Autodesk Inventor part; units mm, degrees
ref_plane "Work Plane1" through (0, 304.8, 0) normal (0, 1, 0) x (-1, 0, 0)
ref_plane "Work Plane2" through (533.4, 247.5686, 0) normal (0, 1, 0) x (-1, 0, 0)
ref_plane "YZ Plane" through (0, 0, 0) normal (1, 0, 0) x (0, 1, 0)
sketch "Sketch1" plane through (0, 0, 0) normal (0, 0, 1) x (1, 0, 0)
  line L0 (0, 0) -> (0, -41.796)
  line L1 (25.4, -16.396) -> (25.4, -41.796)
  arc A0 (0, 0) -> (25.4, -16.396) centre (177.8, 247.5686) ccw
  line L2 (355.6, 0) -> (355.6, -41.796)
  line L3 (330.2, -16.396) -> (330.2, -41.796)
  arc A1 (330.2, -16.396) -> (355.6, 0) centre (177.8, 247.5686) ccw
  line L4 (177.8, 247.5686) -> (533.4, 247.5686)
  line L5 (25.4, -41.796) -> (0, -41.796)
  line L6 (330.2, -41.796) -> (331.8938, -41.796)
  line L7 (331.8938, -41.796) -> (355.6, -41.796)
revolve "Revolution1" add sketch "Sketch1" angle 110 about axis through (177.8, 247.5686, 0) along (1, 0, 0)
sketch "Sketch2" plane through (0, -41.796, 0) normal (0, 0, 1) x (1, 0, 0)
  line L0 (25.4, 0) -> (25.4, 25.4)
  line L1 (355.6, 41.796) -> (355.6, 0)
  arc A0 (330.2, 25.4) -> (355.6, 41.796) centre (177.8, 289.3645) ccw
  line L2 (330.2, 0) -> (330.2, 25.4)
  arc A1 (25.4, 25.4) -> (330.2, 25.4) centre (177.8, 289.3645) ccw
  arc A2 (25.4, 0) -> (330.2, 0) centre (177.8, 263.9645) ccw
  line L3 (25.4, 25.4) -> (25.4, 0)
  line L4 (330.2, 25.4) -> (330.2, 0)
  line L5 (177.8, 289.3645) -> (533.4, 289.3645)
  line L6 (355.6, 0) -> (330.2, 0)
  dimension "d6" = 304.8
  dimension "d7" = 304.8
revolve "Revolution2" add sketch "Sketch2" angle 4 about axis through (177.8, 247.5686, 0) along (1, 0, 0) contours L0 A1 L2 A2
ref_plane "Work Plane1" through (0, 304.8, 0) normal (0, 1, 0) x (-1, 0, 0)
ref_plane "Work Plane2" through (533.4, 247.5686, 0) normal (0, 1, 0) x (-1, 0, 0)
sketch "Sketch8" plane through (533.4, 247.5686, 0) normal (0, 1, 0) x (-1, 0, 0)
  arc A0 (177.8, -247.5686) -> (203.2, -263.9645) centre (355.6, 0) ccw
  line L0 (203.2, -263.9645) -> (203.2, -289.3645)
  line L1 (203.2, -289.3645) -> (177.8, -289.3645)
  line L2 (177.8, -289.3645) -> (177.8, -247.5686)
  line L3 (508, -289.3645) -> (508, -263.9645)
  line L4 (533.4, -247.5686) -> (533.4, -289.3645)
  line L5 (533.4, -289.3645) -> (508, -289.3645)
  arc A1 (203.2, -263.9645) -> (508, -263.9645) centre (355.6, 0) ccw
  arc A2 (203.2, -289.3645) -> (508, -289.3645) centre (355.6, -25.4) ccw
  line L6 (203.2, -289.3645) -> (203.2, -263.9645)
  line L7 (508, -263.9645) -> (508, -289.3645)
  line L8 (355.6, 0) -> (533.4, 0)
  arc A3 (508, -263.9645) -> (533.4, -247.5686) centre (355.6, 0) ccw
  dimension "d44" = 304.8
  dimension "d45" = 304.8
revolve "Revolution4" add sketch "Sketch8" angle 4 about axis through (177.8, 247.5686, 0) along (-1, 0, 0) contours A1 L3 A2 L0
sketch "Sketch9" plane through (25.4, 247.5686, -263.9645) normal (1, 0, 0) x (0, 0, -1)
  line L0 (0, 0) -> (25.4, 0)
  line L1 (-15.919, 90.2812) -> (7.9492, 98.9685)
  line L2 (-3.9849, 94.6248) -> (-3.9849, 81.9248)
  point P0 (-263.9645, -247.5686)
  dimension "d47" = 12.7
hole "Hole3" at (25.4, 329.4934, -259.9796) direction (1, 0, 0) diameter 6.35 end through all
hole "Hole4" at (25.4, 329.4934, -259.9796) direction (-1, 0, 0) diameter 6.35 end through all
sketch "Sketch10" plane through (355.6, -41.796, 0) normal (1, 0, 0) x (0, 0, -1)
  arc A0 (0, 0) -> (271.9137, 388.333) centre (0, 289.3645) ccw
  line L0 (237.0336, 123.3919) -> (467.2357, 16.0468)
  line L1 (165.9727, 52.331) -> (419.9727, 52.331) construction
  line L2 (279.5047, 214.4715) -> (509.7069, 107.1264)
  line L3 (237.0336, 123.3919) -> (491.0336, 123.3919) construction
  line L4 (509.7069, 107.1264) -> (467.2357, 16.0468)
  arc A1 (237.0336, 123.3919) -> (279.5047, 214.4715) centre (0, 289.3645) ccw
  dimension "d65" = 254
  dimension "d66" = 25
  dimension "d67" = 254
  dimension "d68" = 25
extrude "Extrusion3" add sketch "Sketch10" against normal blind 25.4
sketch "Sketch11" plane through (0, -41.796, 0) normal (-1, 0, 0) x (0, 0, 1)
  arc A0 (-271.9137, 388.333) -> (0, 0) centre (0, 289.3645) ccw
  line L0 (-279.5047, 214.4715) -> (-509.7069, 107.1264)
  line L1 (-509.7069, 107.1264) -> (-467.2357, 16.0468)
  line L2 (-467.2357, 16.0468) -> (-237.0336, 123.3919)
extrude "Extrusion4" add sketch "Sketch11" against normal blind 25.4
sketch "Sketch12" plane through (0, -41.796, 0) normal (-1, 0, 0) x (0, 0, 1)
  line L0 (-509.7069, 107.1264) -> (-467.2357, 16.0468)
  line L1 (-467.2357, 16.0468) -> (-237.0336, 123.3919)
  line L2 (-488.4713, 61.5866) -> (-350.35, 125.9937)
  dimension "d73" = 152.4
hole "Hole5" at (0, 84.1977, -350.35) direction (1, 0, 0) diameter 12.7 end through all
sketch "Sketch13" plane through (177.8, 247.5686, -25.4) normal (0, 1, 0) x (1, 0, 0)
  line L0 (152.4, 263.9645) -> (152.4, 238.5645)
  arc A0 (152.4, 238.5645) -> (-152.4, 238.5645) centre (0, -25.4) ccw
  line L1 (152.4, 263.9645) -> (152.4, 352.8645)
  line L2 (152.4, 352.8645) -> (76.2, 352.8645)
  line L3 (76.2, 279.4) -> (76.2, 269.7213)
  line L4 (119.5299, 269.7213) -> (119.5299, 257.7498)
  line L5 (119.5299, 257.7498) -> (152.4, 257.7498)
  line L6 (152.4, 263.9645) -> (152.4, 257.7498)
  line L7 (119.5299, 269.7213) -> (76.2, 269.7213)
  line L8 (-152.4, 238.5645) -> (-152.4, 263.9645)
  line L9 (76.2, 352.8645) -> (0, 352.8645)
  line L10 (0, 352.8645) -> (0, 279.4)
  line L11 (0, 279.4) -> (76.2, 279.4)
  point P0 (-177.8, -25.4)
  dimension "d81" = 88.9
  dimension "d82" = 76.2
  dimension "d85" = 76.2
extrude "Extrusion5" add sketch "Sketch13" against normal blind 18.288 contours L0 L5 L4 L7 L3 L11 L10 L9 L2 L1
sketch "Sketch14" plane through (355.6, -41.796, 0) normal (1, 0, 0) x (0, 0, -1)
  circle A0 centre (350.35, 125.9937) radius 6.35
  circle A1 centre (259.9796, 371.2894) radius 3.175
  line L0 (0, 41.796) -> (0, 0)
  arc A2 (0, 0) -> (237.0336, 123.3919) centre (0, 289.3645) ccw
  line L1 (237.0336, 123.3919) -> (467.2357, 16.0468)
  line L2 (467.2357, 16.0468) -> (509.7069, 107.1264)
  line L3 (509.7069, 107.1264) -> (279.5047, 214.4715)
  arc A3 (279.5047, 214.4715) -> (271.9137, 388.333) centre (0, 289.3645) ccw
  line L4 (232.6384, 374.038) -> (271.9137, 388.333)
  arc A4 (0, 41.796) -> (232.6384, 374.038) centre (0, 289.3645) ccw
  dimension "d86" = 272.5823
properties part number "Inner" material "Polystyrene"
Geometry check sheet. Reference: the model listing, model coordinates, mm. A direction names the side the tool comes from. Round coordinates to 2 decimals unless told otherwise and drop trailing zeros. Order: outer loops, then holes, each group sorted by start corner. A loop starts at its lowest first (then second) coordinate and runs counter-clockwise, first axis right, second up. Notation, with made-up numbers: M 25,7 L 55,7 A20 cw 55,15 Z; hole C -11,-20.75 d4. An arc over 180 degrees is marked long. Write item = value, one per line.
Q1. Depth check by flat-ended pin: pin 1 Ø4 at (y, z) = (329.49, -259.98) entering from +X; pin 2 Ø5.5 at (x, y) = (224, 237) entering from -Z; pin 3 Ø20 at (y, z) = (234.5, -337) entering from +X; pin 4 Ø5.5 at (y, z) = (242, -361.5) entering from -X. Enter the tip coordinate at first touch or a pass-through.
Answer block:
pin_1 = through
pin_2 = -378.26
pin_3 = 330.2
pin_4 = 177.8
Q2. Scan lines: line 1 (X direction, y = -32.5, z = -22.5); line 2 (Y direction, x = 7, z = -350); line 3 (Y direction, x = 256, z = -356). Record each from-to range of solid material in increasing order.
Answer block:
line_1 = 0 to 25.4, 330.2 to 355.6
line_2 = 28.92 to 77.86, 90.54 to 139.8
line_3 = 229.28 to 247.57
Q3. Set-up check for faces 1 (the flat face through (179.93, 225.85, -310.58)), 2 (the flat face through (175.666, -63.011, -21.718)), 3 (the flat face through (330.2, 298, -274)), 4 (the flat face through (12.52, 27.17, -353.75)): record each of +Z, -Z, +X, -X, +Y, -Y from which the full face is reachable in a straight line by a thin tool's end or side.
Answer block:
face_1 = +Z, -Y
face_2 = -Z, +Y
face_3 = +Z, -Z, +Y
face_4 = +X, -X, -Y
Q4. Release check for a two-part mould opening along Z. For faces 5 (the flat face through (12.522, 119.754, -392.994)), 6 (the flat face through (0, 96, -294)), 7 (the cylindrical face through (12.878, 79.906, -355.03)) record: released by +Z, released by -Z, zero draft, split by the parting line, or undercut.
Answer block:
face_5 = released by -Z
face_6 = zero draft
face_7 = undercut
Q5. Section check B-B (z = -419.5). Enter the section's corners in (x, y).
Answer block:
outline = M 0,-3.49 L 25.4,-3.49 L 25.4,107.39 L 0,107.39 Z; M 330.2,-3.49 L 355.6,-3.49 L 355.6,107.39 L 330.2,107.39 Z
Q6. Section check A-A (z = -366.5). Enter the section's corners in (x, y).
Answer block:
outline = M 0,21.22 L 25.4,21.22 L 25.4,132.11 L 0,132.11 Z; M 177.8,229.28 L 330.2,229.28 L 330.2,247.57 L 177.8,247.57 Z; M 330.2,21.22 L 355.6,21.22 L 355.6,132.11 L 330.2,132.11 Z
